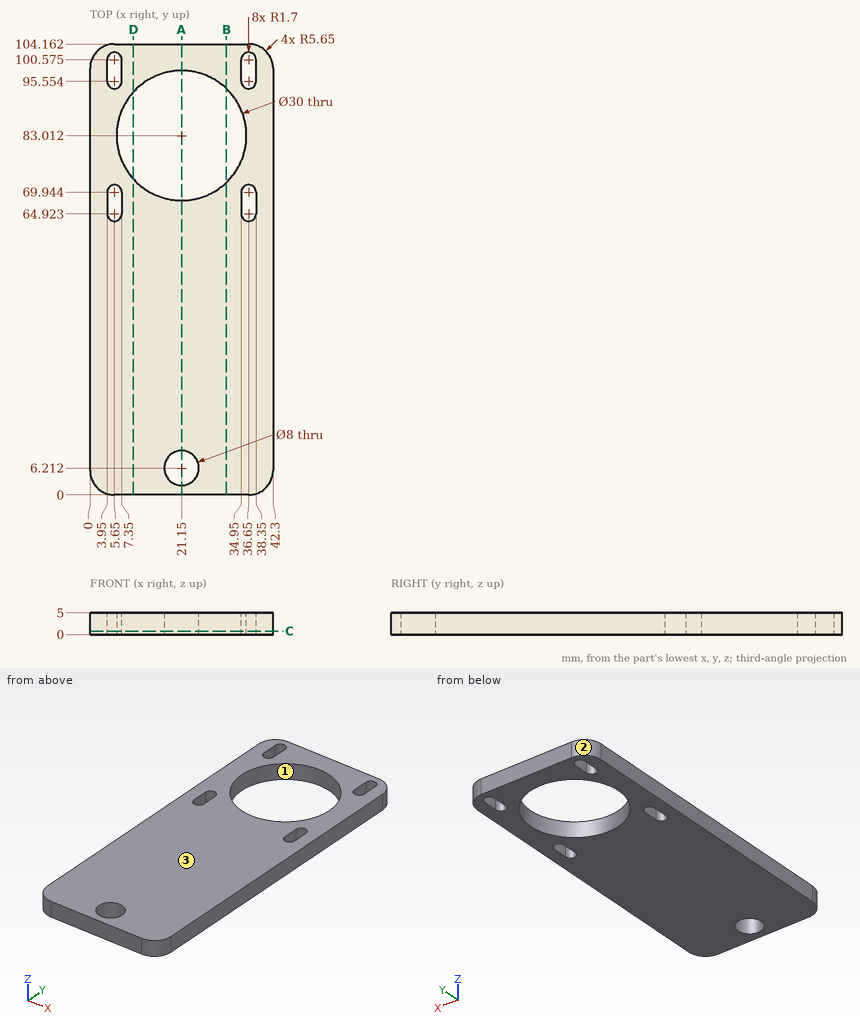
Here's the drawing with two shaded views (mm, measured from the low corner). I have some questions. Coordinates: 2 decimals unless noted, no trailing zeros. Write each loop counter-clockwise with the first axis right and the second up, starting at its lowest first coordinate (ties: lowest second). Pieces come first, ordered by that corner, then holes. Notation, with made-up numbers: (69, 47) - (80, 47) arc R19 cw to (80, 74) - close; hole circle Ø4 at (37.5, -25.75). An arc over 180 degrees is marked (long way). Return JSON: item names as keys, results as strings.
Q1. Please list where these lines run through material, in increasing order: L1, parallel to Y at x = 21.15, z = 2.8; L2, parallel to Y at x = 37, z = 2.2; L3, parallel to X at y = 73, z = 0.7. Write a range as from..to.
Computed values:
{"L1": "y = 0..2.21, 10.21..68.01, 98.01..104.16", "L2": "y = 0.01..63.26, 71.61..93.89, 102.24..104.15", "L3": "x = 0..9.98, 32.32..42.3"}
Q2. If we section it at C-C (z = 0.8): Count the separate pieces of the cut face and the enclosed holes in it, then the cut area to 3 significant figures.
Computed values:
{"separate pieces": "1", "enclosed holes": "6", "area": "3,520 mm2"}
Q3. If we section it at D-D (x = 10): Please give me the cut outline in (y, z).
Computed values:
{"outline": "(0, 0) - (72.98, 0) - (72.98, 5) - (0, 5) - close; (93.05, 0) - (104.16, 0) - (104.16, 5) - (93.05, 5) - close"}
Q4. If we section it at B-B (x = 31.5): Please give me the cut outline in (y, z) (1 decimal), then the cut area to 3 significant figures.
Computed values:
{"outline": "(0, 0) - (72.2, 0) - (72.2, 5) - (0, 5) - close; (93.9, 0) - (104.2, 0) - (104.2, 5) - (93.9, 5) - close", "area": "412 mm2"}
Q5. If we section it at A-A (x = 21.15): Please give me the cut outline in (y, z).
Computed values:
{"outline": "(0, 0) - (2.21, 0) - (2.21, 5) - (0, 5) - close; (10.21, 0) - (68.01, 0) - (68.01, 5) - (10.21, 5) - close; (98.01, 0) - (104.16, 0) - (104.16, 5) - (98.01, 5) - close"}
Q6. I'm going to push a flat-ended pin straight in: pin 1 Ø5 at (x, y) = (14, 91.5) entering from +Z. Where does the tip first touch, or does it pass through?
Computed values:
{"pin 1": "passes through"}
Q7. Thinking about a two-plate mould opening in X: for the marked faces 1, 2 and 3, which applies, +X half, -X half, draft (parallel to the pull), parting line (faces both ways), or undercut?
Computed values:
{"face 1": "undercut", "face 2": "-X half", "face 3": "draft"}
